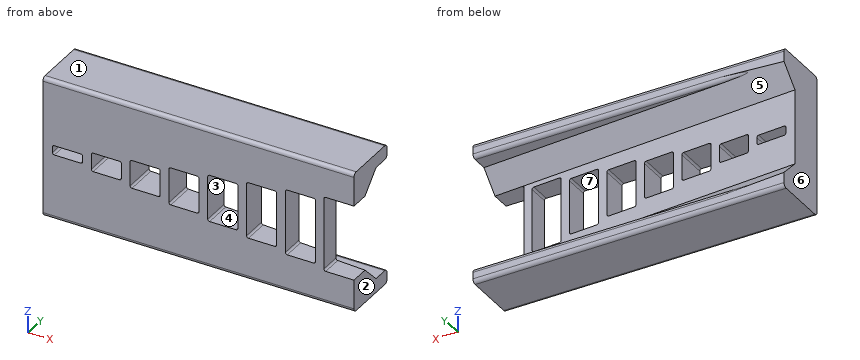
from build123d import *

# Parameters (mm, degrees)
BOSS_EXTRUDE1_DEPTH = 38.1
SKETCH2_W           = 209.55
SKETCH2_H           = 38.1
BOSS_EXTRUDE2_DEPTH = 9.525
SKETCH3_W           = 20.32
SKETCH3_H           = 6.35
SKETCH3_H_2         = 12.7
SKETCH3_H_3         = 19.05
SKETCH3_H_4         = 25.4
SKETCH3_H_5         = 31.75
SKETCH3_H_6         = 38.1
SKETCH3_H_7         = 44.45
SKETCH3_H_8         = 50.8
CUT_EXTRUDE1_DEPTH  = 123.141181515
FILLET1_R           = 1.27
CHAMFER1_SIZE       = 12.7
FILLET2_R           = 2.54


with BuildPart() as part:
    # Sketch1 → Boss-Extrude1 (new, symmetric)
    with BuildSketch(Plane.XY):
        Polygon((-105.823993484, 0), (103.726006516, 0), (103.726006516, 12.7), (-105.823993484, 25.4), align=None)
    extrude(amount=BOSS_EXTRUDE1_DEPTH, both=True)

    # Sketch2 → Boss-Extrude2 (add)
    with BuildSketch(Plane(origin=(0, 0, -38.1), x_dir=(-1, 0, 0), z_dir=(0, 0, -1))):
        with Locations((1.048993484, 19.05)):
            Rectangle(SKETCH2_W, SKETCH2_H)
    boss_extrude2 = extrude(amount=BOSS_EXTRUDE2_DEPTH)

    # Mirror1: Boss-Extrude2 across plane
    add(boss_extrude2.mirror(Plane.XY))

    # Sketch3 → Cut-Extrude1 (cut, through all)
    with BuildSketch(Plane.XZ):
        with Locations((-89.313993484, 0)):
            Rectangle(SKETCH3_W, SKETCH3_H)
        with Locations((-63.151993484, 0)):
            Rectangle(SKETCH3_W, SKETCH3_H_2)
        with Locations((-36.989993484, 0)):
            Rectangle(SKETCH3_W, SKETCH3_H_3)
        with Locations((-10.827993484, 0)):
            Rectangle(SKETCH3_W, SKETCH3_H_4)
        with Locations((15.334006516, 0)):
            Rectangle(SKETCH3_W, SKETCH3_H_5)
        with Locations((41.496006516, 0)):
            Rectangle(SKETCH3_W, SKETCH3_H_6)
        with Locations((67.658006516, 0)):
            Rectangle(SKETCH3_W, SKETCH3_H_7)
        with Locations((93.566006516, 0)):
            Rectangle(SKETCH3_W, SKETCH3_H_8)
    extrude(amount=-CUT_EXTRUDE1_DEPTH, mode=Mode.SUBTRACT)

    # Fillet1
    fillet1_edges = [part.edges().sort_by_distance(p)[0] for p in [
        (-20.987993484, 10.129212121, -12.7),
        (-20.987993484, 10.129212121, 12.7),
        (-0.667993484, 9.513454545, 12.7),
        (-0.667993484, 9.513454545, -12.7),
        (5.174006516, 9.336424242, -15.875),
        (5.174006516, 9.336424242, 15.875),
        (25.494006516, 8.720666667, 15.875),
        (25.494006516, 8.720666667, -15.875),
        (31.336006516, 8.543636364, -19.05),
        (31.336006516, 8.543636364, 19.05),
        (51.656006516, 7.927878788, 19.05),
        (51.656006516, 7.927878788, -19.05),
        (57.498006516, 7.750848485, -22.225),
        (57.498006516, 7.750848485, 22.225),
        (77.818006516, 7.135090909, 22.225),
        (77.818006516, 7.135090909, -22.225),
        (83.406006516, 6.965757576, -25.4),
        (83.406006516, 6.965757576, 25.4),
        (-99.473993484, 12.507575758, 3.175),
        (-79.153993484, 11.891818182, 3.175),
        (-79.153993484, 11.891818182, -3.175),
        (-99.473993484, 12.507575758, -3.175),
        (-73.311993484, 11.714787879, -6.35),
        (-73.311993484, 11.714787879, 6.35),
        (-52.991993484, 11.099030303, 6.35),
        (-52.991993484, 11.099030303, -6.35),
        (-47.149993484, 10.922, -9.525),
        (-47.149993484, 10.922, 9.525),
        (-26.829993484, 10.306242424, 9.525),
        (-26.829993484, 10.306242424, -9.525),
    ]]
    fillet(fillet1_edges, radius=FILLET1_R)

    # Chamfer1
    chamfer1_edges = [part.edges().sort_by_distance(p)[0] for p in [
        (-1.048993484, 19.05, 38.1),
        (-1.048993484, 19.05, -38.1),
    ]]
    chamfer(chamfer1_edges, length=CHAMFER1_SIZE - 0.0001)  # a hair under: the kernel refuses the full size

    # Fillet2
    fillet2_edges = [part.edges().sort_by_distance(p)[0] for p in [
        (-0.85757213, 38.1, -38.1),
        (-1.048993484, 0, -47.625),
        (-1.048993484, 38.1, -47.625),
        (-0.85757213, 38.1, 38.1),
        (-1.048993484, 38.1, 47.625),
        (-1.048993484, 0, 47.625),
    ]]
    fillet(fillet2_edges, radius=FILLET2_R)


solid = part.part
Part model, mm, in its own coordinate system. Face numbers are marked on the shaded views. A direction names the side the tool comes from. Give positions to 0.01 mm unless a question says otherwise; leave off trailing zeros. Order: outer loops, then holes, each group sorted by start corner. A loop starts at its lowest first (then second) coordinate and runs counter-clockwise, first axis right, second up. Notation, with made-up numbers: (12.25, -5.5) -> (30.25, -5.5) arc R23 cw to (30.25, 22.5) -> close; hole circle Ø11 at (-3, 71). An arc over 180 degrees is marked (long way). Use one line per item in the form item = value.
(1) Saw through at C-C (x = -34). Write the cut outline in (y, z) (3 decimals), then the cut area to 3 significant figures.
Solution:
outline = (0, -45.085) arc R2.54 ccw to (2.54, -47.625) -> (35.56, -47.625) arc R2.54 ccw to (38.1, -45.085) -> (38.1, -40.64) arc R2.54 ccw to (35.56, -38.1) -> (33.77, -38.1) -> (21.047, -25.4) -> (21.047, -9.525) -> (0, -9.525) -> close; (0, 9.525) -> (21.047, 9.525) -> (21.047, 25.4) -> (33.77, 38.1) -> (35.56, 38.1) arc R2.54 ccw to (38.1, 40.64) -> (38.1, 45.085) arc R2.54 ccw to (35.56, 47.625) -> (2.54, 47.625) arc R2.54 ccw to (0, 45.085) -> close
area = 2,080 mm²
(2) Flat gauge pins, fed straight in: P1, Ø5, axis at y = 7, z = 0.5, coming from the +X side; P2, Ø3, axis at x = 53.5, z = -18.5, coming from the -Y side. Where does each tip first touch, or does it go through?
Solution:
P1 = 83.41
P2 = 0
(3) Saw through at D-D (z = -32.5). Write the cut outline in (x, y).
Solution:
outline = (-105.82, 0) -> (103.73, 0) -> (103.73, 19.81) -> (-105.82, 32.51) -> close
(4) Saw through at A-A (x = 41). Write the cut outline in (y, z) (3 decimals), then the cut area to 3 significant figures.
Solution:
outline = (0, -45.085) arc R2.54 ccw to (2.54, -47.625) -> (35.56, -47.625) arc R2.54 ccw to (38.1, -45.085) -> (38.1, -40.64) arc R2.54 ccw to (35.56, -38.1) -> (29.225, -38.1) -> (16.502, -25.4) -> (16.502, -19.05) -> (0, -19.05) -> close; (0, 19.05) -> (16.502, 19.05) -> (16.502, 25.4) -> (29.225, 38.1) -> (35.56, 38.1) arc R2.54 ccw to (38.1, 40.64) -> (38.1, 45.085) arc R2.54 ccw to (35.56, 47.625) -> (2.54, 47.625) arc R2.54 ccw to (0, 45.085) -> close
area = 1,510 mm²
(5) Saw through at B-B (y = 30). Write the cut outline in (x, z) (3 decimals), then the cut area to 3 significant figures.
Solution:
outline = (-105.824, -47.625) -> (103.726, -47.625) -> (103.726, -38.1) -> (28.209, -38.1) -> (-105.824, -29.992) -> close; (-105.824, 29.992) -> (28.209, 38.1) -> (103.726, 38.1) -> (103.726, 47.625) -> (-105.824, 47.625) -> close
area = 5,080 mm²
(6) Tool access for the marked faces 5, 6 and 7: list every direction of +Z, -Z, +X, -X, +Y, -Y with a clear straight run to the whole face (end or side of a thin tool).
Solution:
face_5 = +X, +Y
face_6 = +Z, -Z, -X, +Y, -Y
face_7 = +Y, -Y
(7) Pull direction X, two halves, no side cores. Call the marked faces 1, 2, 3 and 4: +X half, -X half, draft (parallel to the pull), parting line (faces both ways), or undercut.
Solution:
face_1 = draft
face_2 = +X half
face_3 = undercut
face_4 = undercut
(8) Drill centre lines: line 1 (Z direction, x = 33, y = 31) (3 decimals); line 2 (Z direction, x = -81, y = 10.5) (3 decimals); line 3 (X direction, y = 21, z = -0.5). Where is each one in solid material? Low to high. Write a range as from..to.
Solution:
line_1 = -47.625..-38.1, 38.1..47.625
line_2 = -47.625..-3.175, 3.175..47.625
line_3 = -105.82..-99.47, -79.15..-73.31, -52.99..-47.15
